Geometry: see drawing. Coordinates: mm, zero at the bounding-box minimum. Round coordinates to 2 decimals unless told otherwise and drop trailing zeros. Loops run counter-clockwise (first coordinate to the right, second up) from the corner with the lowest first, then second, coordinate; pieces in that order, holes last. Notation, with made-up numbers: (-13, -32.75) - (12, -32.75) arc R20 ccw to (12, -15.75) - close; hole circle Ø2 at (-7.5, 83). An arc over 180 degrees is marked (long way). Use CSV: the item, a comma, the result in double quotes.
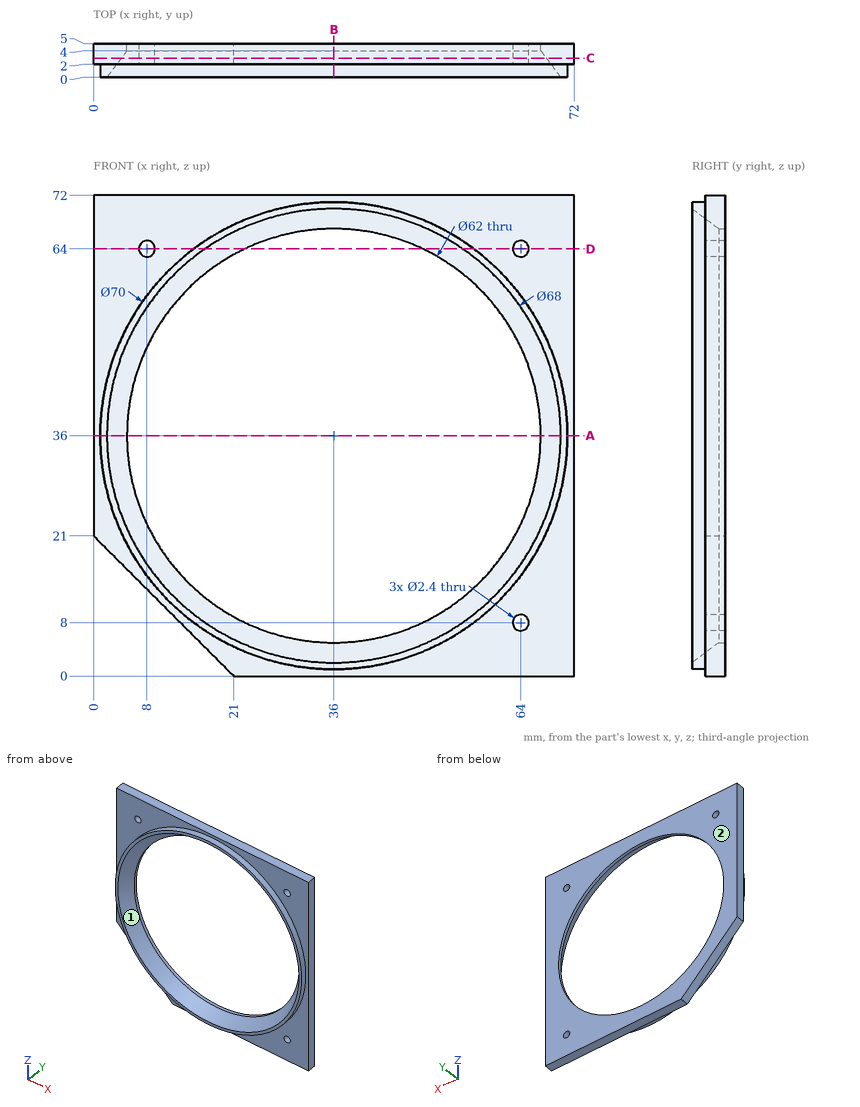
Item 1: Section D-D on z = 64. Give the number of separate pieces and of enclosed holes in the cut face, plus the area to 3 significant figures.
Final values:
separate pieces,"4"
enclosed holes,"0"
area,"128 mm²"
Item 2: Section A-A on z = 36. Return the cut outline in (x, y), plus the area to 3 significant figures.
Final values:
outline,"(0, 2) - (1, 2) - (1, 0) - (2, 0) - (5, 4) - (5, 5) - (0, 5) - close; (67, 4) - (70, 0) - (71, 0) - (71, 2) - (72, 2) - (72, 5) - (67, 5) - close"
area,"34.0 mm²"
Item 3: Material intervals for line 1 (X direction, y = 4.4, z = 36); line 2 (Z direction, x = 64, y = 3), sorted ascending.
Final values:
line 1,"x = 0 to 5, 67 to 72"
line 2,"z = 0 to 6.8, 9.2 to 21.03, 50.97 to 62.8, 65.2 to 72"
Item 4: Section C-C on y = 2.9. Return the cut outline in (x, z) (3 decimals), plus the area to 3 significant figures.
Final values:
outline,"(0, 21) - (21, 0) - (72, 0) - (72, 72) - (0, 72) - close; hole circle Ø63.65 at (36, 36); hole circle Ø2.4 at (8, 64); hole circle Ø2.4 at (64, 8); hole circle Ø2.4 at (64, 64)"
area,"1,770 mm²"
Item 5: Section B-B on x = 36. Return the cut outline in (y, z).
Final values:
outline,"(0, 1) - (2, 1) - (2, 0) - (5, 0) - (5, 5) - (4, 5) - (0, 2) - close; (0, 70) - (4, 67) - (5, 67) - (5, 72) - (2, 72) - (2, 71) - (0, 71) - close"
Item 6: Mould query, pull axis Z, two halves, no side actions, for the marked faces 1 and 2. Classes: released by +Z, released by -Z, zero draft, split by the parting line, or undercut.
Final values:
face 1,"undercut"
face 2,"zero draft"
Item 7: Pin query (flat end, axial travel): P1, Ø2, axis at y = 4, z = 60, coming from the -X side; P2, Ø3, axis at x = 8, z = 64, coming from the -Y side. Return the tip coordinate at first contact, or that it passes through.
Final values:
P1,"stops at x = 0"
P2,"stops at y = 2"
